Check sheet for the drawn part. Datum: minimum x, y, z corner. Units: mm. A direction names the side the tool comes from. Give positions to 0.01 mm unless a question says otherwise; leave off trailing zeros. Write each loop counter-clockwise with the first axis right and the second up, starting at its lowest first coordinate (ties: lowest second). Pieces come first, ordered by that corner, then holes. Notation, with made-up numbers: M -25,60 L -9,60 A9 ccw -9,70 Z; hole C -36.75,46.25 d10. An arc over 180 degrees is marked long. Write item = value, one per line.
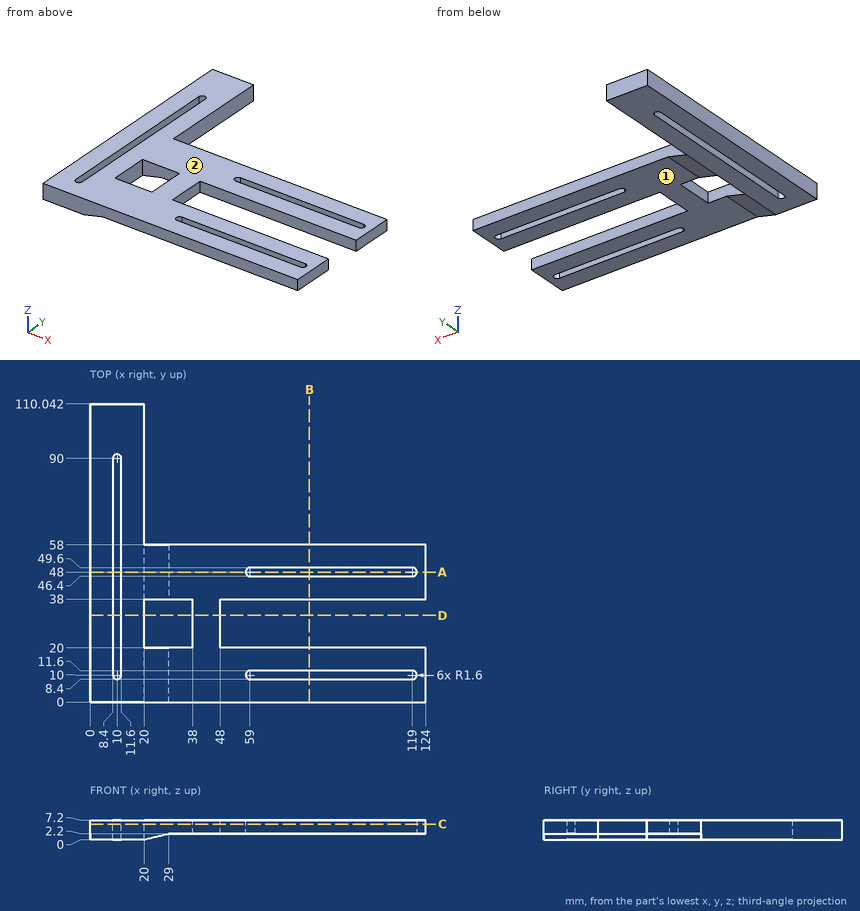
1) Depth check by flat-ended pin: P1, Ø4, axis at y = 97, z = 3, coming from the +X side; P2, Ø1.5, axis at x = 67, z = 5.5, coming from the +Y side; P3, Ø4, axis at y = 25, z = 5, coming from the +X side. Enter the tip coordinate at first touch or a pass-through.
From the geometry:
P1 = 20
P2 = 58
P3 = 48
2) Cross-section at A-A on y = 48. Record the boundary of the cut face in (x, z).
From the geometry:
outline = M 0,0 L 8.4,0 L 8.4,7.2 L 0,7.2 Z; M 11.6,0 L 20,0 L 29,2.2 L 57.4,2.2 L 57.4,7.2 L 11.6,7.2 Z; M 120.6,2.2 L 124,2.2 L 124,7.2 L 120.6,7.2 Z
3) Cross-section at C-C on z = 5.75. Record the boundary of the cut face in (x, y).
From the geometry:
outline = M 0,0 L 124,0 L 124,20 L 48,20 L 48,38 L 124,38 L 124,58 L 20,58 L 20,110.04 L 0,110.04 Z; hole M 8.4,10 A1.6 ccw 11.6,10 L 11.6,90 A1.6 ccw 8.4,90 Z; hole M 20,20 L 38,20 L 38,38 L 20,38 Z; hole M 59,8.4 L 119,8.4 A1.6 ccw 119,11.6 L 59,11.6 A1.6 ccw Z; hole M 59,46.4 L 119,46.4 A1.6 ccw 119,49.6 L 59,49.6 A1.6 ccw Z
4) Cross-section at B-B on x = 81. Record the boundary of the cut face in (y, z), plus the area to 3 significant figures.
From the geometry:
outline = M 0,2.2 L 8.4,2.2 L 8.4,7.2 L 0,7.2 Z; M 11.6,2.2 L 20,2.2 L 20,7.2 L 11.6,7.2 Z; M 38,2.2 L 46.4,2.2 L 46.4,7.2 L 38,7.2 Z; M 49.6,2.2 L 58,2.2 L 58,7.2 L 49.6,7.2 Z
area = 168 mm^2
5) Cross-section at D-D on y = 32. Record the boundary of the cut face in (x, z), plus the area to 3 significant figures.
From the geometry:
outline = M 0,0 L 8.4,0 L 8.4,7.2 L 0,7.2 Z; M 11.6,0 L 20,0 L 20,7.2 L 11.6,7.2 Z; M 38,2.2 L 48,2.2 L 48,7.2 L 38,7.2 Z
area = 171 mm^2
6) Tool access check on the marked faces 1 and 2. Record the directions out of +Z, -Z, +X, -X, +Y, -Y that give a thin tool (end or side, any length) a straight path to the whole face; none if there is none.
From the geometry:
face_1 = -Z, +X, +Y, -Y
face_2 = +Z, +X, -X, +Y, -Y
7) Material ranges on probe 1 along Y at (x, z) = (66, 4); probe 2 along X at (y, z) = (82, 0.5); probe 3 along X at (y, z) = (18.5, 5.5), recorded low to high. Write a range as from..to.
From the geometry:
probe_1 = 0..8.4, 11.6..20, 38..46.4, 49.6..58
probe_2 = 0..8.4, 11.6..20
probe_3 = 0..8.4, 11.6..124
